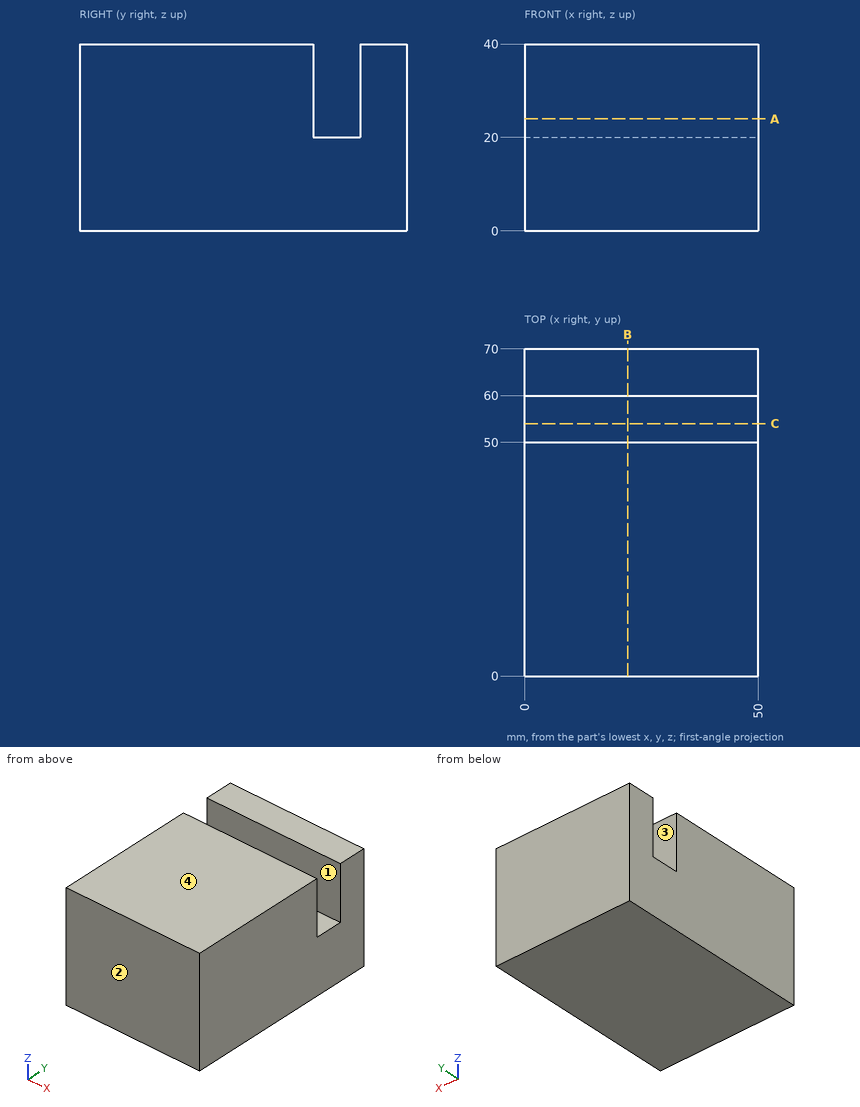
Job drawing, mm, ordinate dimensions from the low corner. One solid piece. Coordinates: 2 decimals unless noted, no trailing zeros. Write each loop counter-clockwise with the first axis right and the second up, starting at its lowest first coordinate (ties: lowest second). Pieces come first, ordered by that corner, then holes.
Item 1: Mould opens along Y. For the marked faces 1, 2, 3 and 4 say: released by +Y, released by -Y, zero draft, split by the parting line, or undercut.
Item 2: Slice it at A-A (z = 24). Write the cut outline in (x, y).
Item 3: Probe line 1 (Y direction, x = 22, z = 28.5); line 2 (Z direction, x = 15, y = 51.5). List the from-to ranges inside material, lowest first.
Item 4: Pin check, flat tips, straight feed: pin 1 (1.5 mm diameter, centred on x = 16, y = 37.5, fed in from -Z); pin 2 (5 mm diameter, centred on x = 13.5, y = 56, fed in from +Z). Stop position of each tip, or through.
Item 5: Slice it at B-B (x = 22). Write the cut outline in (y, z), and give its area (3 significant figures).
Item 6: Slice it at C-C (y = 54). Write the cut outline in (x, z), and give its area (3 significant figures).
Results found:
1. face 1: undercut
1. face 2: released by -Y
1. face 3: undercut
1. face 4: zero draft
2. outline: (0, 0) - (50, 0) - (50, 50) - (0, 50) - close; (0, 60) - (50, 60) - (50, 70) - (0, 70) - close
3. line 1: y = 0 to 50, 60 to 70
3. line 2: z = 0 to 20
4. pin 1: stops at z = 0
4. pin 2: stops at z = 20
5. outline: (0, 0) - (70, 0) - (70, 40) - (60, 40) - (60, 20) - (50, 20) - (50, 40) - (0, 40) - close
5. area: 2,600 mm2
6. outline: (0, 0) - (50, 0) - (50, 20) - (0, 20) - close
6. area: 1,000 mm2
